Part model, mm, in its own coordinate system. A direction names the side the tool comes from. Coordinates: 2 decimals unless noted, no trailing zeros. Order: outer loops, then holes, each group sorted by start corner. A loop starts at its lowest first (then second) coordinate and runs counter-clockwise, first axis right, second up.
from build123d import *

# Parameters (mm, degrees)
F0_W        = 30
F0_H        = 10
F1_DEPTH    = 10
F2_R        = 5
F3_T1_DEPTH = 84.348882825
F4_R        = 10
F5_R        = 50
F6_SIZE     = 2
F8_DEPTH    = 10.001
F9_SIZE     = 2
F10_DEPTH   = 16
F11_DEPTH   = 25


# Not quite as in the source:
# - a fillet or chamfer that OpenCascade refuses, or shapes differently, is made with other operations: its cross-section is extruded or revolved along the edge and cut away or added


with BuildPart() as f1:
    # F0 (on Top) → F1 (new body)
    with BuildSketch(Plane.XY):
        Polygon((5, 50), (-5, 50), (-15, 65), (-15, 75), (-25, 75), (-25, 61.9722436227), (-5, 31.9722436227), (-5, -50), (5, -50), (5, 31.9722436227), (25, 61.9722436227), (25, 75), (15, 75), (15, 65), align=None)
        with Locations((0, 70)):
            Rectangle(F0_W, F0_H)
    extrude(amount=F1_DEPTH)

    # F2
    f2_edges = [f1.edges().sort_by_distance(p)[0] for p in [
        (15, 65, 5),
        (-15, 65, 5),
        (-5, 50, 5),
        (5, 50, 5),
    ]]
    fillet(f2_edges, radius=F2_R)

    # F3: fillet of radius 15 on 2 edges, made by hand

    # F3_s2 → F3_t1 (cut)
    with BuildSketch(Plane.XY.offset(-37.1744414125)):
        with BuildLine():
            ThreePointArc((-25, 61.9722436227), (-20.0149678844, 71.2823679771), (-10.130223435, 75))
            Line((-10.130223435, 75), (-25, 75))
            Line((-25, 75), (-25, 61.9722436227))
        make_face()
        with BuildLine():
            ThreePointArc((25, 61.9722436227), (20.0149678844, 71.2823679771), (10.130223435, 75))
            Line((10.130223435, 75), (25, 75))
            Line((25, 75), (25, 61.9722436227))
        make_face()
    extrude(amount=F3_T1_DEPTH, mode=Mode.SUBTRACT)

    # F4
    f4_edges = [f1.edges().sort_by_distance(p)[0] for p in [
        (-25, 61.972244, 5),
        (25, 61.972244, 5),
    ]]
    fillet(f4_edges, radius=F4_R)

    # F5
    f5_edges = [f1.edges().sort_by_distance(p)[0] for p in [
        (5, 31.972244, 5),
        (-5, 31.972244, 5),
    ]]
    fillet(f5_edges, radius=F5_R)

    # F6
    f6_edges = [f1.edges().sort_by_distance(p)[0] for p in [
        (0, 65, 10),
        (0, 75, 10),
        (0, 50, 0),
        (0, 75, 0),
    ]]
    chamfer(f6_edges, length=F6_SIZE)

    # F7 (on face) → F8 (cut, through all)
    with BuildSketch(Plane.XY.offset(10)):
        Polygon((0, 37.3431457505), (2.8284271247, 40.1715728753), (0, 43), (-2.8284271247, 40.1715728753), align=None)
    extrude(amount=-F8_DEPTH, mode=Mode.SUBTRACT)

    # F9
    f9_edges = [f1.edges().sort_by_distance(p)[0] for p in [
        (1.414214, 41.585786, 10),
        (-1.414214, 41.585786, 10),
        (1.414214, 38.757359, 10),
        (-1.414214, 38.757359, 10),
        (1.414214, 38.757359, 0),
        (1.414214, 41.585786, 0),
        (-1.414214, 41.585786, 0),
        (-1.414214, 38.757359, 0),
    ]]
    chamfer(f9_edges, length=F9_SIZE)

    # F10 (add): a face of the model
    f10_faces = [f1.faces().sort_by_distance(p)[0] for p in [
        (0, -50, 5),
    ]]
    extrude(f10_faces, amount=-F10_DEPTH)

    # F11 (cut): a face of the model
    f11_faces = [f1.faces().sort_by_distance(p)[0] for p in [
        (0, -50, 5),
    ]]
    extrude(f11_faces, amount=-F11_DEPTH, mode=Mode.SUBTRACT)


solid = f1.part
Q1. Mould opens along X. For faces 1 (the face through (-7.2, 31.5, 5)), 2 (the face through (0, 50, 5)), 3 (the face through (-2, 46, 0)), 4 (the face through (1.394, 38.738, 5.042)) say: pulls with the +X half, pulls with the -X half, needs draft (parallel to the pull), parting line crosses it, or undercut.
Results list:
face 1: pulls with the -X half
face 2: undercut
face 3: needs draft
face 4: undercut
Q2. Cut at B-B on y = -15.5. Write the cut outline in (x, z).
Results list:
outline: (-5, 2) - (-3, 0) - (3, 0) - (5, 2) - (5, 8) - (3, 10) - (-3, 10) - (-5, 8) - close
Q3. Cut at A-A on z = 5.5. Write the cut outline in (x, y), and give its area (3 significant figures).
Results list:
outline: (-22.2, 57.77) - (-13.4, 44.57) arc R50 cw to (-5, 16.83) - (-5, -25) - (5, -25) - (5, 16.83) arc R50 cw to (13.4, 44.57) - (22.2, 57.77) arc R10 ccw to (21.37, 69.94) arc R15 ccw to (10.13, 75) - (-10.13, 75) arc R15 ccw to (-21.37, 69.94) arc R10 ccw to start; hole (-9.82, 57.23) - (-6.48, 52.23) arc R5 ccw to (-2.32, 50) - (2.32, 50) arc R5 ccw to (6.48, 52.23) - (9.82, 57.23) arc R5 ccw to (5.66, 65) - (-5.66, 65) arc R5 ccw to start; hole (-2.83, 40.17) - (0, 37.34) - (2.83, 40.17) - (0, 43) - close
area: 1,790 mm2
Q4. Which spindle directions (+Z, -Z, +X, -X, +Y, -Y) get a long thin tool onto all of the face, cutting with end or side? Do faces 5 (the face through (2.23, 37.86, 0.79)), 6 (the face through (4, -4, 9)), 7 (the face through (-1, 42, 5)), 8 (the face through (-2.2, 42.5, 9.2)), 9 (the face through (-23.845, 64.085, 5.042)). Say none if no direction does.
Results list:
face 5: -Z
face 6: +Z, +X, -Y
face 7: +Z, -Z
face 8: +Z
face 9: +Z, -Z, -X
Q5. Pin check, flat tips, straight feed: pin 1 Ø3 at (x, z) = (-6.5, 9) entering from +Y; pin 2 Ø3 at (y, z) = (42, 2.5) entering from +X; pin 3 Ø3 at (y, z) = (1.5, 3.5) entering from -X. Stop position of each tip, or through.
Results list:
pin 1: stops at y = 75
pin 2: stops at x = 12.7
pin 3: stops at x = -5
Q6. Wall check: line 1 along X through (y, z) = (65, 9.5); line 2 along Y through (x, z) = (-1.5, 8.5); line 3 along X through (y, z) = (-10, 6). Give the ranges that are in metal, low to high.
Results list:
line 1: x = -22.21 to -9.81, 9.81 to 22.21
line 2: y = -25 to 38.14, 42.21 to 49.5, 65.5 to 74.5
line 3: x = -5 to 5
